Design review of the part built by this model. Coordinates are the model's own, in mm. Coordinates: 2 decimals unless noted, no trailing zeros. Order: outer loops, then holes, each group sorted by start corner. A loop starts at its lowest first (then second) coordinate and runs counter-clockwise, first axis right, second up. Notation, with made-up numbers: M -1,45 L 17,45 A24 ccw 17,71 Z; hole C 40,54 d2. An arc over 180 degrees is marked long. Use CSV: the item, a comma, the result in double quotes.
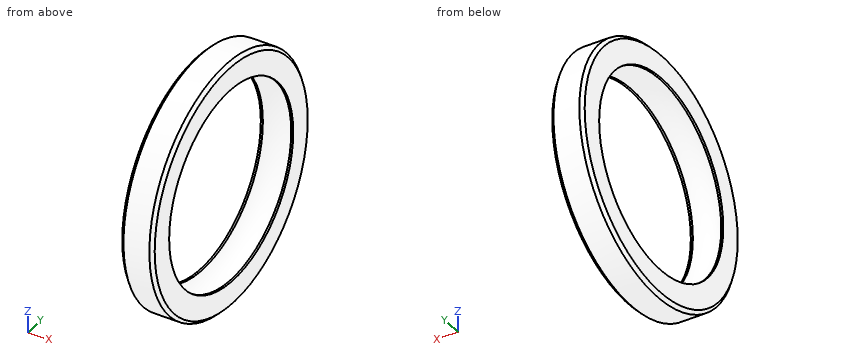
```python
from build123d import *

# Parameters (mm, degrees)
CHAMFER2_SIZE = 0.5


with BuildPart() as part:
    # Sketch1 → Revolve2 (revolve)
    with BuildSketch(Plane.XY):
        with BuildLine():
            Line((-2.5, 15), (-2.188493664, 15))
            ThreePointArc((-2.188493664, 15), (0, 15.948050809), (2.188493664, 15))
            Line((2.188493664, 15), (2.5, 15))
            Line((2.5, 15), (2.5, 19))
            Line((2.5, 19), (-2.5, 19))
            Line((-2.5, 19), (-2.5, 15))
        make_face()
    revolve(axis=Axis((-21.395056223, 0, 0), (1, 0, 0)))

    # Chamfer2
    chamfer2_edges = [part.edges().sort_by_distance(p)[0] for p in [
        (-2.5, -19, 0),
        (2.5, -19, 0),
    ]]
    chamfer(chamfer2_edges, length=CHAMFER2_SIZE)


solid = part.part
```
(1) Add section D-D on x = 1.15. State the section outline as (y, z) points, and give its area (3 significant figures).
The answers:
outline,"C 0,0 d38; hole C 0,0 d31.44"
area,"358 mm2"
(2) Wall thickness on probe 1 along Z at (x, y) = (2.35, 0); probe 2 along Z at (x, y) = (2.45, 0); probe 3 along Y at (x, z) = (0.8, -3.5): over which ranges is each line inside the solid? List them lowest first.
The answers:
probe 1,"z = -18.65 to -15, 15 to 18.65"
probe 2,"z = -18.55 to -15, 15 to 18.55"
probe 3,"y = -18.67 to -15.45, 15.45 to 18.67"
(3) Add section A-A on y = 0. State the section outline as (x, z) points.
The answers:
outline,"M -2.5,-18.5 L -2,-19 L 2,-19 L 2.5,-18.5 L 2.5,-15 L 2.19,-15 A3 cw -2.19,-15 L -2.5,-15 Z; M -2.5,15 L -2.19,15 A3 cw 2.19,15 L 2.5,15 L 2.5,18.5 L 2,19 L -2,19 L -2.5,18.5 Z"
(4) Clearance check with flat-ended pins moving along their axes: P1, Ø3, axis at x = 2, y = -10.5, coming from the +Z side; P2, Ø2, axis at x = -1.5, y = -1, coming from the +Z side. State where each tip first meets the part, or that it passes through.
The answers:
P1,"stops at z = 16.73"
P2,"stops at z = 19"
(5) Add section C-C on x = -0.9. State the section outline as (y, z) points, and give its area (3 significant figures).
The answers:
outline,"C 0,0 d38; hole C 0,0 d31.62"
area,"349 mm2"
